from build123d import *

# Parameters (mm, degrees)
F0_W     = 240
F0_H     = 165
F1_DEPTH = 30
F2_T     = -2
F3_SIZE  = 5


with BuildPart() as f1:
    # F0 (on Top) → F1 (new body)
    with BuildSketch(Plane.XY):
        Rectangle(F0_W, F0_H)
    extrude(amount=F1_DEPTH)

    # F2
    f2_openings = [f1.faces().sort_by_distance(p)[0] for p in [
        (0, 0, 30),
    ]]
    offset(amount=F2_T, openings=f2_openings)

    # F3
    f3_edges = [f1.edges().sort_by_distance(p)[0] for p in [
        (-118, 80.5, 16),
        (118, 80.5, 16),
        (-118, -80.5, 16),
        (118, -80.5, 16),
        (120, -82.5, 15),
        (120, 82.5, 15),
        (-120, -82.5, 15),
        (-120, 82.5, 15),
        (120, 0, 0),
        (0, 82.5, 0),
        (-120, 0, 0),
        (0, -82.5, 0),
        (118, 0, 2),
        (0, 80.5, 2),
        (-118, 0, 2),
        (0, -80.5, 2),
    ]]
    chamfer(f3_edges, length=F3_SIZE)


solid = f1.part
Design review of the part built by this model. Coordinates are the model's own, in mm. A direction names the side the tool comes from. Give positions to 0.01 mm unless a question says otherwise; leave off trailing zeros. Loops run counter-clockwise (first coordinate to the right, second up) from the corner with the lowest first, then second, coordinate; pieces in that order, holes last. Notation, with made-up numbers: (-36.5, 28) - (-18.5, 28) arc R13 cw to (-18.5, 44) - close; hole circle Ø3 at (60, 80.25). An arc over 180 degrees is marked (long way). Use CSV: the item, a comma, the result in double quotes. Start each with the question number.
1. Draft analysis for pull direction X (two halves, no side actions). For faces 3 (the flat face through (-116.5, 79.1, 3.1)), 4 (the flat face through (-114.5, 77.1, 5.1)), 5 (the flat face through (-1.6, -78, 4.5)), 6 (the flat face through (-2, 82.5, 17)), state which applies: released by +X, released by -X, zero draft, split by the parting line, or undercut.
2. Insertion check: P1, Ø2, axis at x = 50, y = 54.5, coming from the +Z side. The pin has a flat end and moves straight along its axis. Give the tip position at first contact, or say it passes through.
3. Add section A-A (z = 14.5). State the section outline as (x, y) points.
4. Add section C-C (y = -32). State the section outline as (x, z) points, plus the area to 3 significant figures.
5. Machinability: for faces 1 (the flat face through (-2, 1, 2)), 2 (the flat face through (-1.6, 80, 2.5)), which of the approach directions +Z, -Z, +X, -X, +Y, -Y give a long, thin tool a straight path to every point of the face, cutting with its end or side? Answer none if there is none.
6. Add section B-B (x = -63). State the section outline as (y, z) points, plus the area to 3 significant figures.
7. Wall thickness on L1, parallel to X at y = -32.5, z = 11; L2, parallel to Y at x = -85, z = 8.75; L3, parallel to Z at x = 57, y = 9.5: over which ranges is each line inside the solid? List them lowest first.
Results found:
1,face 3,"released by -X"
1,face 4,"undercut"
1,face 5,"undercut"
1,face 6,"zero draft"
2,P1,"stops at z = 2"
3,outline,"(-120, -77.5) - (-115, -82.5) - (115, -82.5) - (120, -77.5) - (120, 77.5) - (115, 82.5) - (-115, 82.5) - (-120, 77.5) - close; hole (-118, -75.5) - (-113, -80.5) - (113, -80.5) - (118, -75.5) - (118, 75.5) - (113, 80.5) - (-113, 80.5) - (-118, 75.5) - close"
4,outline,"(-120, 5) - (-115, 0) - (115, 0) - (120, 5) - (120, 30) - (118, 30) - (118, 7) - (113, 2) - (-113, 2) - (-118, 7) - (-118, 30) - (-120, 30) - close"
4,area,"592 mm²"
5,face 1,"+Z"
5,face 2,"-Z, +X, -X, +Y"
6,outline,"(-82.5, 5) - (-77.5, 0) - (77.5, 0) - (82.5, 5) - (82.5, 30) - (80.5, 30) - (80.5, 7) - (75.5, 2) - (-75.5, 2) - (-80.5, 7) - (-80.5, 30) - (-82.5, 30) - close"
6,area,"442 mm²"
7,L1,"x = -120 to -118, 118 to 120"
7,L2,"y = -82.5 to -80.5, 80.5 to 82.5"
7,L3,"z = 0 to 2"
